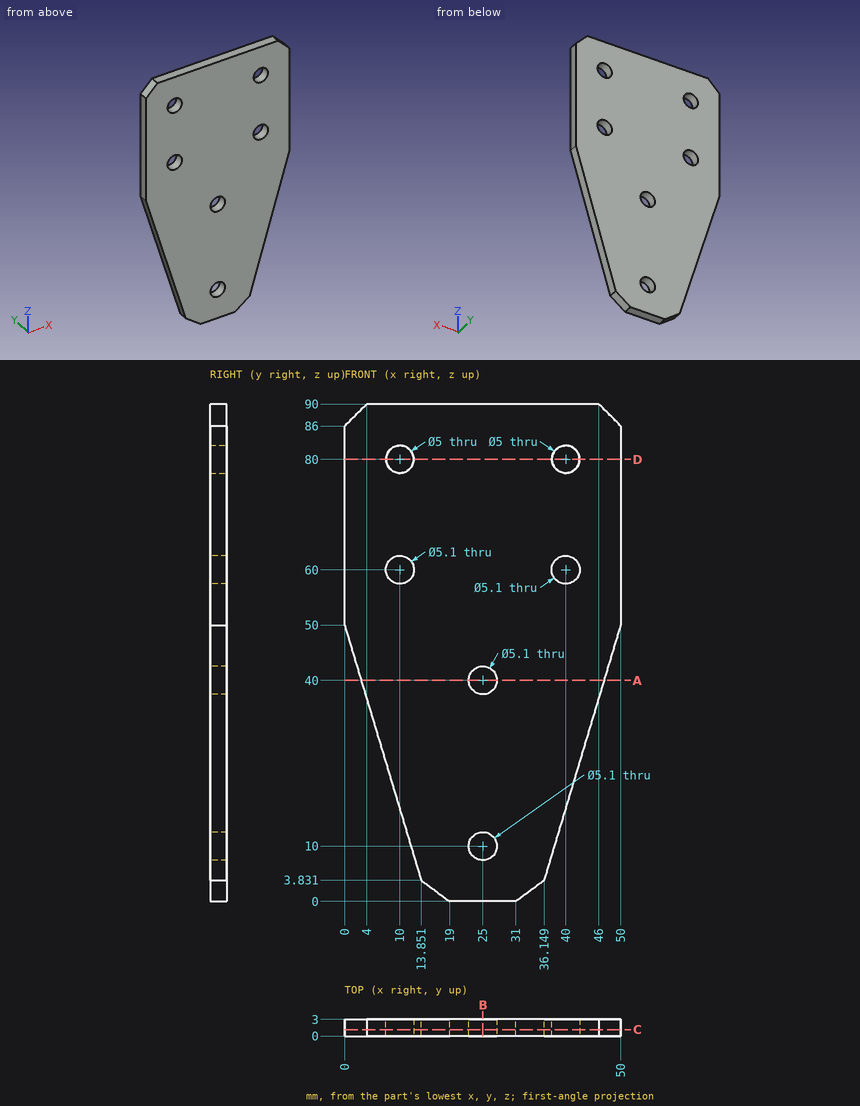
The drawing under review shows one solid part. Ordinate dimensions are in mm from its lowest x, y, z. Coordinates: 2 decimals unless noted, no trailing zeros. Loops run counter-clockwise (first coordinate to the right, second up) from the corner with the lowest first, then second, coordinate; pieces in that order, holes last.
Item 1: Add section D-D (z = 80). Write out the cut boundary in (x, y), and give its area (3 significant figures).
Completed:
outline: (0, 0) - (7.5, 0) - (7.5, 3) - (0, 3) - close; (12.5, 0) - (37.5, 0) - (37.5, 3) - (12.5, 3) - close; (42.5, 0) - (50, 0) - (50, 3) - (42.5, 3) - close
area: 120 mm2
Item 2: Wall thickness on L1, parallel to X at y = 1.05, z = 80; L2, parallel to Z at x = 25.5, y = 2.85; L3, parallel to Z at x = 24, y = 2.4 (1 decimal): over which ranges is each line inside the solid? List them lowest first.
Completed:
L1: x = 0 to 7.5, 12.5 to 37.5, 42.5 to 50
L2: z = 0 to 7.5, 12.5 to 37.5, 42.5 to 90
L3: z = 0 to 7.7, 12.3 to 37.7, 42.3 to 90
Item 3: Add section C-C (y = 1.15). Write out the cut boundary in (x, z), and give its area (3 significant figures).
Completed:
outline: (0, 50) - (13.85, 3.83) - (19, 0) - (31, 0) - (36.15, 3.83) - (50, 50) - (50, 86) - (46, 90) - (4, 90) - (0, 86) - close; hole circle Ø5.1 at (10, 60); hole circle Ø5 at (10, 80); hole circle Ø5.1 at (25, 10); hole circle Ø5.1 at (25, 40); hole circle Ø5.1 at (40, 60); hole circle Ø5 at (40, 80)
area: 3,600 mm2
Item 4: Clearance check with flat-ended pins moving along their axes: pin 1 (1.5 mm diameter, centred on y = 1.5, z = 19.5, fed in from +X) (1 decimal); pin 2 (1 mm diameter, centred on y = 1, z = 39, fed in from +X); pin 3 (1 mm diameter, centred on y = 1.5, z = 14, fed in from +X). State where each tip first meets the part, or that it passes through.
Completed:
pin 1: stops at x = 41.1
pin 2: stops at x = 46.85
pin 3: stops at x = 39.35
Item 5: Add section B-B (x = 25). Write out the cut boundary in (y, z).
Completed:
outline: (0, 0) - (3, 0) - (3, 7.45) - (0, 7.45) - close; (0, 12.55) - (3, 12.55) - (3, 37.45) - (0, 37.45) - close; (0, 42.55) - (3, 42.55) - (3, 90) - (0, 90) - close
Item 6: Add section A-A (z = 40). Write out the cut boundary in (x, y).
Completed:
outline: (3, 0) - (22.45, 0) - (22.45, 3) - (3, 3) - close; (27.55, 0) - (47, 0) - (47, 3) - (27.55, 3) - close
